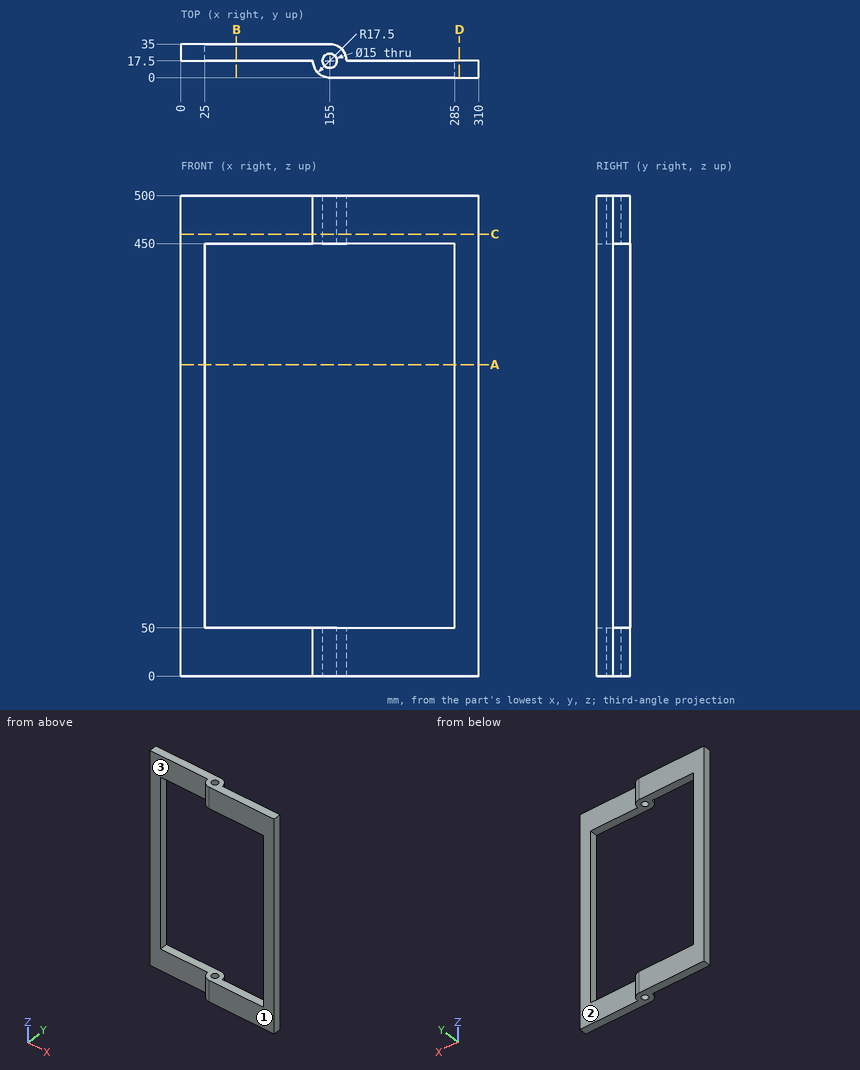
Check sheet for the drawn part. Datum: minimum x, y, z corner. Units: mm. A direction names the side the tool comes from. Round coordinates to 2 decimals unless told otherwise and drop trailing zeros. Loops run counter-clockwise (first coordinate to the right, second up) from the corner with the lowest first, then second, coordinate; pieces in that order, holes last. Notation, with made-up numbers: (52, -35.5) - (99, -35.5) arc R16 ccw to (99, -29.5) - close; hole circle Ø4 at (4, 80). An arc over 180 degrees is marked (long way). Use one line per item in the form item = value.
1. Gauge pin test, flat ends, axial feed: pin 1 Ø1 at (y, z) = (15.5, 151.5) entering from -X; pin 2 Ø6 at (y, z) = (26.5, 380) entering from +X; pin 3 Ø5 at (x, y) = (254.5, 18) entering from -Z. Record the tip position at first contact, or that the pin passes through.
A:
pin_1 = 285
pin_2 = 25
pin_3 = 0
2. Section check B-B on x = 58. Record the cut outline in (y, z), and give its area (3 significant figures).
A:
outline = (17.5, 0) - (35, 0) - (35, 50) - (17.5, 50) - close; (17.5, 450) - (35, 450) - (35, 500) - (17.5, 500) - close
area = 1,750 mm²
3. Section check A-A on z = 324. Record the cut outline in (x, y).
A:
outline = (0, 17.5) - (25, 17.5) - (25, 35) - (0, 35) - close; (285, 0) - (310, 0) - (310, 17.5) - (285, 17.5) - close
4. Scan lines: probe 1 along Z at (x, y) = (284, 14); probe 2 along X at (y, z) = (17, 25); probe 3 along Y at (x, z) = (155, 17). Record each from-to range of solid material in increasing order.
A:
probe_1 = 0 to 50, 450 to 500
probe_2 = 137.51 to 147.52, 162.48 to 310
probe_3 = 0 to 10, 25 to 35
5. Access from +Z, -Z, +X, -X, +Y, -Y to the whole of each face (thin tool, end or side, straight path). Record for the marked faces 1, 2 and 3.
A:
face_1 = +Z, -Z, +X, -X, -Y
face_2 = +Z, -Z, +X, +Y
face_3 = +Z, -Z, -X, -Y
6. Section check C-C on z = 460. Record the cut outline in (x, y).
A:
outline = (0, 17.5) - (137.5, 17.5) arc R17.5 ccw to (155, 0) - (310, 0) - (310, 17.5) - (172.5, 17.5) arc R17.5 ccw to (155, 35) - (0, 35) - close; hole circle Ø15 at (155, 17.5)
7. Section check D-D on x = 290. Record the cut outline in (y, z).
A:
outline = (0, 0) - (17.5, 0) - (17.5, 500) - (0, 500) - close
